Part model, mm, in its own coordinate system. Round coordinates to 2 decimals unless told otherwise and drop trailing zeros. Loops run counter-clockwise (first coordinate to the right, second up) from the corner with the lowest first, then second, coordinate; pieces in that order, holes last. Notation, with made-up numbers: (65, 57.5) -> (86, 57.5) arc R10 cw to (86, 67.5) -> close; hole circle Ø7 at (41, 23.5). An arc over 180 degrees is marked (long way). Use a Markdown table: item, result. Add a question column.
Item 1: Cut at C-C, the plane y = 6.5. List the corners of the cut face in (x, z).
Item 2: Cut at B-B, the plane x = -11. List the corners of the cut face in (y, z).
Item 3: Probe line 1 (Y direction, x = -1, z = 0.7); line 2 (Y direction, x = 13.5, z = 1.4); line 3 (X direction, y = -27, z = 0.85). List the from-to ranges inside material, lowest first. Write a range as [from, to].
Item 4: Cut at A-A, the plane z = 0.75. List the corners of the cut face in (x, y).
Item 5: Flat gauge pins, fed straight in: pin 1 (5 mm diameter, centred on x = 15.2, y = 23.98, fed in from -Z) (3 decimals); pin 2 (6.5 mm diameter, centred on x = -38.49, y = -33.02, fed in from -Z). Where does each tip first touch, or does it go through?
```python
from build123d import *

# Parameters (mm, degrees)
F0_R     = 2
F1_DEPTH = 1.5
F2_SIZE  = 1


with BuildPart() as f1:
    # F0 (on Top) → F1 (new body)
    with BuildSketch(Plane.XY):
        with BuildLine():
            Line((-9.189322, 27.726636), (-44.985039, -34.273364))
            ThreePointArc((-44.985039, -34.273364), (-44.985039, -36.773364), (-42.819975, -38.023364))
            Line((-42.819975, -38.023364), (-16.261863, -38.023364))
            ThreePointArc((-16.261863, -38.023364), (-15.011863, -37.688427), (-14.096799, -36.773364))
            Line((-14.096799, -36.773364), (21.698917, 25.226636))
            ThreePointArc((21.698917, 25.226636), (21.698917, 27.726636), (19.533854, 28.976636))
            Line((19.533854, 28.976636), (-7.024259, 28.976636))
            ThreePointArc((-7.024259, 28.976636), (-8.274259, 28.6417), (-9.189322, 27.726636))
        make_face()
        with Locations((-38.489848, -33.023364)):
            Circle(F0_R, mode=Mode.SUBTRACT)
        with Locations((15.203727, 23.976636)):
            Circle(F0_R, mode=Mode.SUBTRACT)
    extrude(amount=F1_DEPTH)

    # F2
    f2_edges = [f1.edges().sort_by_distance(p)[0] for p in [
        (13.203727, 23.976636, 0),
        (-40.489848, -33.023364, 0),
    ]]
    chamfer(f2_edges, length=F2_SIZE)


solid = f1.part
```
A:
| question | item | result |
|---|---|---|
| 1 | outline | (-21.44, 0) -> (10.89, 0) -> (10.89, 1.5) -> (-21.44, 1.5) -> close |
| 2 | outline | (-31.41, 0) -> (24.59, 0) -> (24.59, 1.5) -> (-31.41, 1.5) -> close |
| 3 | line 1 | y = [-14.09, 28.98] |
| 3 | line 2 | y = [11.03, 22.93], [25.02, 28.98] |
| 3 | line 3 | x = [-40.79, -8.45] |
| 4 | outline | (-44.99, -34.27) arc R2.5 ccw to (-42.82, -38.02) -> (-16.26, -38.02) arc R2.5 ccw to (-14.1, -36.77) -> (21.7, 25.23) arc R2.5 ccw to (19.53, 28.98) -> (-7.02, 28.98) arc R2.5 ccw to (-9.19, 27.73) -> close; hole circle Ø4.5 at (-38.49, -33.02); hole circle Ø4.5 at (15.2, 23.98) |
| 5 | pin 1 | stops at z = 0.495 |
| 5 | pin 2 | stops at z = 0 |
